The figure shows three views and two pictorial views of one solid part (mm, origin at its lowest corner). Answer the questions. A direction names the side the tool comes from. Coordinates: 2 decimals unless noted, no trailing zeros. Order: outer loops, then holes, each group sorted by start corner. A loop starts at its lowest first (then second) coordinate and runs counter-clockwise, first axis right, second up. Notation, with made-up numbers: M -30.5,56.5 L -4.5,56.5 A33 cw -4.5,87.5 Z; hole C 18.5,48.25 d5. An arc over 180 degrees is marked long. Answer in a Markdown table with one row per item. Add a question column.
Item 1: The part is cut by section C-C (z = 35). Write down the section's boundary in (x, y).
Item 2: Flat-ended cylindrical pins translate along their axes: pin 1 Ø8 at (x, z) = (36.5, 26) entering from -Y; pin 2 Ø4 at (x, y) = (76.5, 19.5) entering from +Z; pin 3 Ø3 at (y, z) = (8.5, 6) entering from -X; pin 4 Ø5 at (x, y) = (44.5, 29.5) entering from +Z. Find the tip coordinate at first contact, or state that the pin passes through.
Item 3: Consider line 1 (Y direction, x = 19.5, z = 32); line 2 (Z direction, x = 14, y = 22). Determine where each line is inside the solid, lowest interval first. Write a range as from..to.
Item 4: The part is cut by section A-A (x = 12.5). Write down the section's boundary in (y, z), then the cut area to 3 significant figures.
Item 5: The part is cut by section B-B (y = 25). Write down the section's boundary in (x, z).
Item 6: Which of the six approach directions +Z, -Z, +X, -X, +Y, -Y give full straight-line access (tool end or side, diameter ignored) to the marked faces 1 and 2?
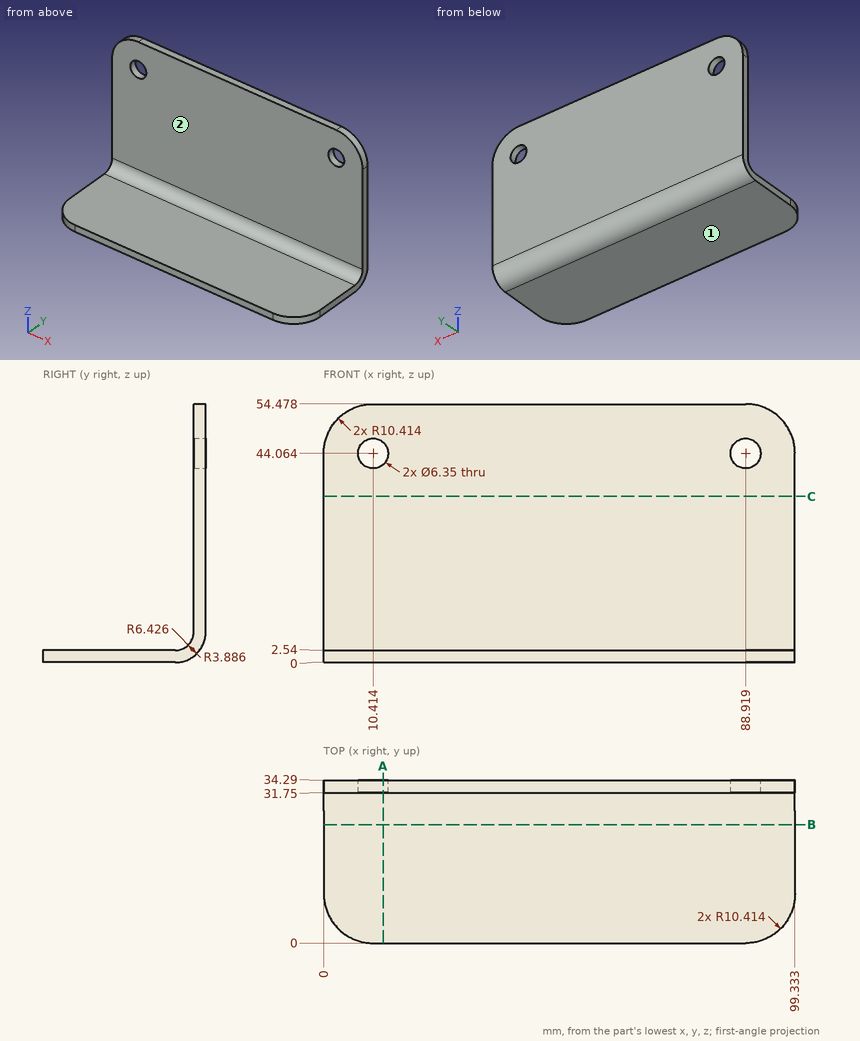
Reply:
| question | item | result |
|---|---|---|
| 1 | outline | M 0,31.75 L 99.33,31.75 L 99.33,34.29 L 0,34.29 Z |
| 2 | pin 1 | stops at y = 31.75 |
| 2 | pin 2 | stops at z = 2.54 |
| 2 | pin 3 | passes through |
| 2 | pin 4 | stops at z = 54.48 |
| 3 | line 1 | y = 31.75..34.29 |
| 3 | line 2 | z = 0..2.54 |
| 4 | outline | M 0,0 L 27.86,0 A6.43 ccw 34.29,6.43 L 34.29,41.67 L 31.75,41.67 L 31.75,6.43 A3.89 cw 27.86,2.54 L 0,2.54 Z; M 31.75,46.46 L 34.29,46.46 L 34.29,54.48 L 31.75,54.48 Z |
| 4 | area | 201 mm2 |
| 5 | outline | M 0,0 L 99.33,0 L 99.33,2.54 L 0,2.54 Z |
| 6 | face 1 | -Z, +X, -X, +Y, -Y |
| 6 | face 2 | +Z, +X, -X, -Y |
